from build123d import *

# Parameters (mm, degrees)
F1_DEPTH = 914.4


with BuildPart() as f1:
    # F0 (on Top) → F1 (new body)
    with BuildSketch(Plane.XY):
        with BuildLine():
            Line((76.2, 355.6), (-76.2, 355.6))
            ThreePointArc((-76.2, 355.6), (-104.742894, 193.193469), (-114.3, 28.575002))
            add(Edge.make_bspline(
                [(-95.25, 57.15), (-114.299999, 57.15), (-114.3, 28.575002)],
                knots=[0, 0, 0, 1.570796, 1.570796, 1.570796], degree=2, weights=[1, 0.707107, 1]))
            add(Edge.make_bspline(
                [(-95.25, 0), (-76.2, 0), (-76.2, 28.575), (-76.2, 57.15), (-95.25, 57.15)],
                knots=[3.141593, 3.141593, 3.141593, 4.712389, 4.712389, 6.283185, 6.283185, 6.283185], degree=2, weights=[1, 0.707107, 1, 0.707107, 1]))
            Line((-95.25, 0), (95.25, 0))
            add(Edge.make_bspline(
                [(95.25, 57.15), (76.2, 57.15), (76.2, 28.575), (76.2, 0), (95.25, 0)],
                knots=[0, 0, 0, 1.570796, 1.570796, 3.141593, 3.141593, 3.141593], degree=2, weights=[1, 0.707107, 1, 0.707107, 1]))
            add(Edge.make_bspline(
                [(114.3, 28.575), (114.3, 57.15), (95.25, 57.15)],
                knots=[4.712389, 4.712389, 4.712389, 6.283185, 6.283185, 6.283185], degree=2, weights=[1, 0.707107, 1]))
            ThreePointArc((114.3, 28.575), (104.742894, 193.193468), (76.2, 355.6))
        make_face()
        with BuildLine():
            add(Edge.make_bspline(
                [(-95.25, 57.15), (-114.299999, 57.15), (-114.3, 28.575002)],
                knots=[0, 0, 0, 1.570796, 1.570796, 1.570796], degree=2, weights=[1, 0.707107, 1]))
            add(Edge.make_bspline(
                [(-114.3, 28.575002), (-114.300001, 0), (-95.25, 0)],
                knots=[1.570796, 1.570796, 1.570796, 3.141593, 3.141593, 3.141593], degree=2, weights=[1, 0.707107, 1]))
            add(Edge.make_bspline(
                [(-95.25, 0), (-76.2, 0), (-76.2, 28.575), (-76.2, 57.15), (-95.25, 57.15)],
                knots=[3.141593, 3.141593, 3.141593, 4.712389, 4.712389, 6.283185, 6.283185, 6.283185], degree=2, weights=[1, 0.707107, 1, 0.707107, 1]))
        make_face()
        with BuildLine():
            add(Edge.make_bspline(
                [(95.25, 0), (114.3, 0), (114.3, 28.575)],
                knots=[3.141593, 3.141593, 3.141593, 4.712389, 4.712389, 4.712389], degree=2, weights=[1, 0.707107, 1]))
            add(Edge.make_bspline(
                [(114.3, 28.575), (114.3, 57.15), (95.25, 57.15)],
                knots=[4.712389, 4.712389, 4.712389, 6.283185, 6.283185, 6.283185], degree=2, weights=[1, 0.707107, 1]))
            add(Edge.make_bspline(
                [(95.25, 57.15), (76.2, 57.15), (76.2, 28.575), (76.2, 0), (95.25, 0)],
                knots=[0, 0, 0, 1.570796, 1.570796, 3.141593, 3.141593, 3.141593], degree=2, weights=[1, 0.707107, 1, 0.707107, 1]))
        make_face()
    extrude(amount=F1_DEPTH)


solid = f1.part
Design review of the part built by this model. Coordinates are the model's own, in mm. Give positions to 0.01 mm unless a question says otherwise; leave off trailing zeros. Write each loop counter-clockwise with the first axis right and the second up, starting at its lowest first coordinate (ties: lowest second). Pieces come first, ordered by that corner, then holes. Notation, with made-up numbers: M 39.5,-25 L 75.5,-25 A17 cw 75.5,1 Z; hole C 9,44.5 d6. An arc over 180 degrees is marked long. Answer as a JSON object with one key per item and string values. Group by question number.
1) We need section A-A (y = 148). Give the boundary of the cut face in (x, z), and give its area (3 significant figures).
2) Clearance check with flat-ended pins moving along their axes: pin 1 Ø1 at (y, z) = (243.5, 313) entering from +X; pin 2 Ø5 at (x, z) = (-85.5, 423) entering from -Y. State where each tip first meets the part, or that it passes through.
3) We need section B-B (x = -86). Give the boundary of the cut face in (y, z).
4) For line 1 along X through (y, z) = (28, 60); line 2 along X through (y, z) = (98.5, 123), list the stretches that pass through material, from the lowest coordinate up.
Answer key:
{
 "1": {"outline": "M -109.28,0 L 109.28,0 L 109.28,914.4 L -109.28,914.4 Z", "area": "200,000 mm²"},
 "2": {"pin 1": "stops at x = 98.05", "pin 2": "stops at y = 0"},
 "3": {"outline": "M 0,0 L 310.91,0 L 310.91,914.4 L 0,914.4 Z"},
 "4": {"line 1": "x = -114.3 to 114.3", "line 2": "x = -112.58 to 112.58"}
}
